The listing builds one solid part. Answer for the finished solid, in the listing's coordinates (mm). Face numbers are marked on the shaded views. A direction names the side the tool comes from. Coordinates: 2 decimals unless noted, no trailing zeros. Order: outer loops, then holes, each group sorted by start corner. A loop starts at its lowest first (then second) coordinate and runs counter-clockwise, first axis right, second up. Notation, with made-up numbers: (-33, 24.25) -> (-9, 24.25) arc R15 ccw to (-9, 41.25) -> close; hole circle Ø1 at (39, 5). An arc over 180 degrees is marked (long way). Return JSON: item names as keys, results as strings.
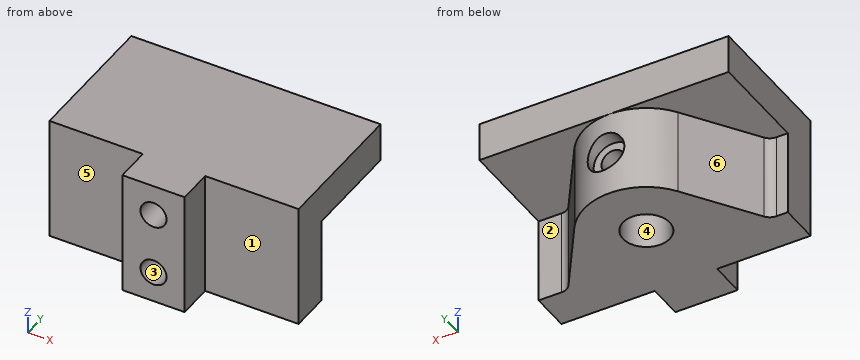
```python
from build123d import *

# Parameters (mm, degrees)
SKETCH2_R           = 6
BOSS_EXTRUDE1_DEPTH = 11
SKETCH3_W           = 64
SKETCH3_H           = 36
BOSS_EXTRUDE2_DEPTH = 10
BOSS_EXTRUDE3_DEPTH = 32
SKETCH5_R           = 5
CUT_EXTRUDE5_DEPTH  = 4
SKETCH7_R           = 3
CUT_EXTRUDE6_DEPTH  = 10


with BuildPart() as part:
    # Sketch2 → Boss-Extrude1 (new, symmetric)
    with BuildSketch(Plane.XY):
        with BuildLine():
            Line((-30.479384134, -10), (-27.579076202, -10))
            ThreePointArc((-27.579076202, -10), (-26.167523045, -9.647171639), (-25.087993879, -8.671678457))
            Line((-25.087993879, -8.671678457), (-13.285772387, 8.915618436))
            ThreePointArc((-13.285772387, 8.915618436), (-0.796428366, 15.98016589), (12.333454196, 10.192443652))
            Line((12.333454196, 10.192443652), (13.285772387, 8.915618436))
            Line((13.285772387, 8.915618436), (25.087993879, -8.671678457))
            ThreePointArc((25.087993879, -8.671678457), (26.167523045, -9.647171639), (27.579076202, -10))
            Line((27.579076202, -10), (30.479384134, -10))
            Line((30.479384134, -10), (31.075959419, -10))
            Line((31.075959419, -10), (33.520615866, -10))
            Line((33.520615866, -10), (33.520615866, -20))
            Line((33.520615866, -20), (-30.479384134, -20))
            Line((-30.479384134, -20), (-30.479384134, -10))
        make_face()
        Circle(SKETCH2_R, mode=Mode.SUBTRACT)
    extrude(amount=BOSS_EXTRUDE1_DEPTH, both=True)

    # Sketch3 → Boss-Extrude2 (add)
    with BuildSketch(Plane.XY.offset(11)):
        with Locations((1.520615866, -2)):
            Rectangle(SKETCH3_W, SKETCH3_H)
    extrude(amount=BOSS_EXTRUDE2_DEPTH)

    # Sketch4 → Boss-Extrude3 (add)
    with BuildSketch(Plane(origin=(0, 0, -11), x_dir=(-1, 0, 0), z_dir=(0, 0, -1))):
        Polygon((-1.520615866, -20), (6.479384134, -20), (6.479384134, -29), (-9.520615866, -29), (-9.520615866, -20), align=None)
    extrude(amount=-BOSS_EXTRUDE3_DEPTH)

    # Sketch5 → Cut-Extrude5 (cut)
    with BuildSketch(Plane(origin=(0, 16, 0), x_dir=(1, 0, 0), z_dir=(0, 1, 0))):
        with Locations(Location((1.520615866, -1, 0), (0, 0, 270))):
            Circle(SKETCH5_R)
    extrude(amount=-CUT_EXTRUDE5_DEPTH, mode=Mode.SUBTRACT)

    # Sketch7 → Cut-Extrude6 (cut)
    with BuildSketch(Plane(origin=(0, 12, 0), x_dir=(1, 0, 0), z_dir=(0, 1, 0))):
        with Locations(Location((1.520615866, -1, 0), (0, 0, 270))):
            Circle(SKETCH7_R)
    extrude(amount=-CUT_EXTRUDE6_DEPTH, mode=Mode.SUBTRACT)

    # Sketch11 → Cut-Revolve1 (revolve, cut)
    with BuildSketch(Plane(origin=(1.520615866, 0, 0), x_dir=(0, 0, -1), z_dir=(1, 0, 0))):
        Polygon((3, -29), (3, -13), (3, -11.065876598), (6.35, -13), (6.35, -29), align=None)
    revolve(axis=Axis((1.520615866, -13, -3), (0, 1, 0)), mode=Mode.SUBTRACT)

    # Sketch14 → Cut-Revolve2 (revolve, cut)
    with BuildSketch(Plane(origin=(1.520615866, 0, 0), x_dir=(0, 0, -1), z_dir=(1, 0, 0)), mode=Mode.PRIVATE) as cut_revolve2_sk:
        Polygon((-16.35, -29), (-13, -29), (-13, -11.065876598), (-16.35, -13), align=None)
    revolve(cut_revolve2_sk.sketch.rotate(Axis((1.520615866, -29, 13), (0, 1, 0)), 180), axis=Axis((1.520615866, -29, 13), (0, 1, 0)), mode=Mode.SUBTRACT)


solid = part.part
```
Item 1: Determine the mould class of the marked faces 4, 5 and 6 for opening direction Y: pulls with the +Y half, pulls with the -Y half, needs draft (parallel to the pull), parting line crosses it, or undercut.
Answer list:
{"face 4": "undercut", "face 5": "pulls with the -Y half", "face 6": "pulls with the +Y half"}
Item 2: The part is cut by section C-C on y = 0. Determine the outline of the cut face in (x, z).
Answer list:
{"outline": "(-30.48, 11) -> (-19.27, 11) -> (-19.27, -11) -> (-6, -11) -> (-6, 11) -> (6, 11) -> (6, -11) -> (19.27, -11) -> (19.27, 11) -> (33.52, 11) -> (33.52, 21) -> (-30.48, 21) -> close"}
Item 3: The part is cut by section D-D on x = 21. Determine the outline of the cut face in (y, z).
Answer list:
{"outline": "(-20, -11) -> (-2.58, -11) -> (-2.58, 11) -> (16, 11) -> (16, 21) -> (-20, 21) -> close"}
Item 4: Find the intervals of material crossed by probe 1 along X at (y, z) = (-26.5, 11.5); probe 2 along X at (y, z) = (-23, -3); probe 3 along Z at (x, y) = (2, -3), in increasing order.
Answer list:
{"probe 1": "-6.48 to -1.47, 4.52 to 9.52", "probe 2": "-6.48 to -1.83, 4.87 to 9.52", "probe 3": "11 to 21"}
Item 5: The part is cut by section A-A on y = -21. Determine the outline of the cut face in (x, z), plus the area to 3 significant figures.
Answer list:
{"outline": "(-6.48, -11) -> (9.52, -11) -> (9.52, 21) -> (-6.48, 21) -> close; hole circle Ø6.7 at (1.52, -3); hole circle Ø6.7 at (1.52, 13)", "area": "441 mm2"}
Item 6: The part is cut by section B-B on x = -23. Determine the outline of the cut face in (y, z).
Answer list:
{"outline": "(-20, -11) -> (-5.56, -11) -> (-5.56, 11) -> (16, 11) -> (16, 21) -> (-20, 21) -> close"}
Item 7: Flat-ended cylindrical pins translate along their axes: pin 1 (1.8 mm diameter, centred on x = 31, z = -2, fed in from +Y); pin 2 (11 mm diameter, centred on x = 0, y = 0, fed in from -Z); pin 3 (5 mm diameter, centred on x = 13, z = 11, fed in from -Y). Find the tip coordinate at first contact, or state that the pin passes through.
Answer list:
{"pin 1": "y = -10", "pin 2": "z = 11", "pin 3": "y = -20"}
Item 8: Which of the six approach directions +Z, -Z, +X, -X, +Y, -Y give full straight-line access (tool end or side, diameter ignored) to the marked faces 1, 2 and 3?
Answer list:
{"face 1": "+Z, -Z, +X, -Y", "face 2": "-Z, +X, +Y", "face 3": "-Y"}
